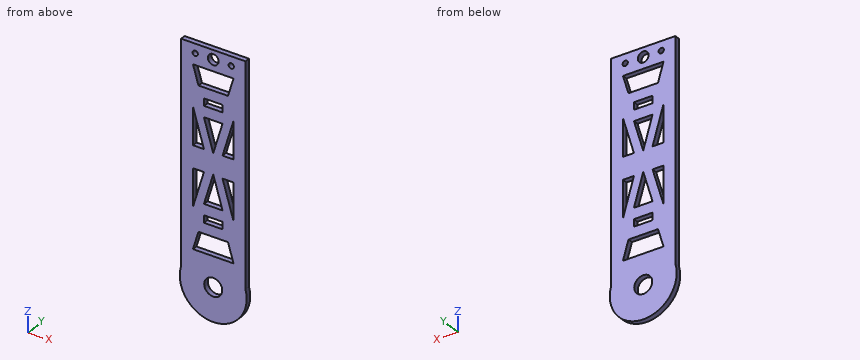
```python
from build123d import *

# Parameters (mm, degrees)
BOSS_EXTRUDE1_DEPTH     = 2
SKETCH5_W               = 3.614771896
SKETCH5_H               = 2.818898279
CUT_EXTRUDE4_DEPTH      = 2
MIRROR3_COPY_1_SKETCH_W = 3.614771896
MIRROR3_COPY_1_SKETCH_H = 2.818898279
MIRROR3_COPY_1_DEPTH    = 2
SKETCH6_R               = 3.5
CUT_EXTRUDE5_DEPTH      = 3
CUT_EXTRUDE5_DEPTH_BACK = 1
CUT_EXTRUDE7_REACH      = 4
SKETCH8_R               = 2.084098117
SKETCH8_R_2             = 1.022428323


with BuildPart() as part:
    # Sketch2 → Boss-Extrude1 (new body)
    with BuildSketch(Plane(origin=(0, 0, 0), x_dir=(1, 0, 0), z_dir=(0, 1, 0))):
        with BuildLine():
            Line((-12.5, -42.5), (12.5, -42.5))
            Line((12.5, -42.5), (12.5, 42.5))
            ThreePointArc((12.5, 42.5), (0, 59.070714214), (-12.5, 42.5))
            Line((-12.5, 42.5), (-12.5, -42.5))
        make_face()
    extrude(amount=BOSS_EXTRUDE1_DEPTH)

    # Sketch5 → Cut-Extrude4 (cut)
    with BuildSketch(Plane(origin=(0, 0, 0), x_dir=(1, 0, 0), z_dir=(0, 1, 0))):
        Polygon((0, 34.507006909), (7.873050165, 34.507006909), (5.742382303, 27.303155751), (0, 27.303155751), align=None)
        with Locations((1.807385948, 21.821964654)):
            Rectangle(SKETCH5_W, SKETCH5_H)
        Polygon((0, 16.184168096), (3.614771896, 16.184168096), (0, 3.962517237), align=None)
        Polygon((7.873050165, 18.689855455), (3.614771896, 4.28215314), (7.873050165, 4.28215314), align=None)
    cut_extrude4 = extrude(amount=CUT_EXTRUDE4_DEPTH, mode=Mode.SUBTRACT)

    # Mirror1: Cut-Extrude4 across plane
    add(cut_extrude4.mirror(Plane(origin=(0, 0, 0), x_dir=(0, 0, 1), z_dir=(1, 0, 0))), mode=Mode.SUBTRACT)

    # Mirror3: Cut-Extrude4 across plane
    add(cut_extrude4.mirror(Plane.XY), mode=Mode.SUBTRACT)

    # Mirror3 copy 1 sketch → Mirror3 copy 1 (cut)
    with BuildSketch(Plane(origin=(0, 0, 0), x_dir=(-1, 0, 0), z_dir=(0, 1, 0))):
        Polygon((0, 34.507006909), (7.873050165, 34.507006909), (5.742382303, 27.303155751), (0, 27.303155751), align=None)
        with Locations((1.807385948, 21.821964654)):
            Rectangle(MIRROR3_COPY_1_SKETCH_W, MIRROR3_COPY_1_SKETCH_H)
        Polygon((0, 16.184168096), (3.614771896, 16.184168096), (0, 3.962517237), align=None)
        Polygon((7.873050165, 18.689855455), (3.614771896, 4.28215314), (7.873050165, 4.28215314), align=None)
    extrude(amount=MIRROR3_COPY_1_DEPTH, mode=Mode.SUBTRACT)

    # Sketch6 → Cut-Extrude5 (cut, two sides)
    with BuildSketch(Plane(origin=(0, 0, 0), x_dir=(1, 0, 0), z_dir=(0, 1, 0))) as cut_extrude5_sk:
        with Locations((0, 46.070714214)):
            Circle(SKETCH6_R)
    extrude(amount=CUT_EXTRUDE5_DEPTH, mode=Mode.SUBTRACT)
    extrude(cut_extrude5_sk.sketch, amount=-CUT_EXTRUDE5_DEPTH_BACK, mode=Mode.SUBTRACT)

    # Sketch8 → Cut-Extrude7 (cut, up to next)
    with BuildSketch(Plane(origin=(0, 0, 0), x_dir=(1, 0, 0), z_dir=(0, 1, 0)), mode=Mode.PRIVATE) as cut_extrude7_sk1:
        with Locations((0, -38.904058143)):
            Circle(SKETCH8_R)
    cut_extrude7_tool1 = extrude(cut_extrude7_sk1.sketch, amount=CUT_EXTRUDE7_REACH, mode=Mode.PRIVATE) & part.part
    add(cut_extrude7_tool1.solids().sort_by_distance((0, 0, 38.904058))[0], mode=Mode.SUBTRACT)
    # Sketch8 → Cut-Extrude7 (cut, up to next)
    with BuildSketch(Plane(origin=(0, 0, 0), x_dir=(1, 0, 0), z_dir=(0, 1, 0)), mode=Mode.PRIVATE) as cut_extrude7_sk2:
        with Locations((7, -38.904058143)):
            Circle(SKETCH8_R_2)
    cut_extrude7_tool2 = extrude(cut_extrude7_sk2.sketch, amount=CUT_EXTRUDE7_REACH, mode=Mode.PRIVATE) & part.part
    add(cut_extrude7_tool2.solids().sort_by_distance((7, 0, 38.904058))[0], mode=Mode.SUBTRACT)
    # Sketch8 → Cut-Extrude7 (cut, up to next)
    with BuildSketch(Plane(origin=(0, 0, 0), x_dir=(1, 0, 0), z_dir=(0, 1, 0)), mode=Mode.PRIVATE) as cut_extrude7_sk3:
        with Locations((-7, -38.904058143)):
            Circle(SKETCH8_R_2)
    cut_extrude7_tool3 = extrude(cut_extrude7_sk3.sketch, amount=CUT_EXTRUDE7_REACH, mode=Mode.PRIVATE) & part.part
    add(cut_extrude7_tool3.solids().sort_by_distance((-7, 0, 38.904058))[0], mode=Mode.SUBTRACT)


solid = part.part
```
Part model, mm, in its own coordinate system. Give positions to 0.01 mm unless a question says otherwise; leave off trailing zeros. Write each loop counter-clockwise with the first axis right and the second up, starting at its lowest first coordinate (ties: lowest second). Pieces come first, ordered by that corner, then holes. Notation, with made-up numbers: (-14, 11) -> (26, 11) arc R7 ccw to (26, 16) -> close; hole circle Ø9 at (76, 38.25). An arc over 180 degrees is marked (long way). Put each result on its own line as item: value. Start each with the question number.
Item 1: Cut at C-C (z = -2.5). List the corners of the cut face in (x, y).
Item 2: Wall check: L1, parallel to X at y = 0.35, z = 14; L2, parallel to X at y = 1.35, z = -40; L3, parallel to X at y = 1.25, z = -6. Give the ranges that are in metal, low to high. Write a range as [from, to].
Item 3: Cut at A-A (z = 10). List the corners of the cut face in (x, y).
Item 4: Cut at B-B (x = 7). List the corners of the cut face in (y, z), then the cut area to 3 significant figures.
Item 5: Cut at D-D (y = 0.9). State how many separate pieces and enclosed holes the cut face has, then the cut area to 3 significant figures.
Item 6: Pin check, flat tips, straight feed: pin 1 Ø0.6 at (x, y) = (-2.5, 1) entering from -Z; pin 2 Ø1 at (x, z) = (-7.5, 15) entering from -Y; pin 3 Ø1 at (x, y) = (8.5, 0) entering from -Z; pin 4 Ø0.6 at (x, y) = (1, 1) entering from -Z. Stop position of each tip, or through.
Answer list:
1. outline: (-12.5, 0) -> (12.5, 0) -> (12.5, 2) -> (-12.5, 2) -> close
2. L1: x = [-12.5, -7.87], [-6.49, -2.97], [2.97, 6.49], [7.87, 12.5]
2. L2: x = [-12.5, 12.5]
2. L3: x = [-12.5, -7.87], [-4.12, -0.6], [0.6, 4.12], [7.87, 12.5]
3. outline: (-12.5, 0) -> (-7.87, 0) -> (-7.87, 2) -> (-12.5, 2) -> close; (-5.3, 0) -> (-1.79, 0) -> (-1.79, 2) -> (-5.3, 2) -> close; (1.79, 0) -> (5.3, 0) -> (5.3, 2) -> (1.79, 2) -> close; (7.87, 0) -> (12.5, 0) -> (12.5, 2) -> (7.87, 2) -> close
4. outline: (0, -57.03) -> (2, -57.03) -> (2, -34.51) -> (0, -34.51) -> close; (0, -31.56) -> (2, -31.56) -> (2, -15.74) -> (0, -15.74) -> close; (0, -4.28) -> (2, -4.28) -> (2, 4.28) -> (0, 4.28) -> close; (0, 15.74) -> (2, 15.74) -> (2, 31.56) -> (0, 31.56) -> close; (0, 34.51) -> (2, 34.51) -> (2, 37.88) -> (0, 37.88) -> close; (0, 39.93) -> (2, 39.93) -> (2, 42.5) -> (0, 42.5) -> close
4. area: 137 mm2
5. separate pieces: 1
5. enclosed holes: 14
5. area: 1,980 mm2
6. pin 1: stops at z = -58.88
6. pin 2: stops at y = 0
6. pin 3: stops at z = -56.32
6. pin 4: stops at z = -59.05
